Input: part model. Units: mm. Frame: model coordinates. Round coordinates to 2 decimals unless told otherwise and drop trailing zeros. Order: outer loops, then holes, each group sorted by start corner. A loop starts at its lowest first (then second) coordinate and runs counter-clockwise, first axis right, second up.
Item 1: Cut plane B-B on y = -22.5. Output: boundary loops of the cut face in (x, z).
Item 2: Cut plane C-C on z = 4.5. Output: boundary loops of the cut face in (x, y), then the cut area to 3 significant figures.
Item 3: Cut plane A-A on z = 0. Output: boundary loops of the cut face in (x, y).
Item 4: Line query: L1, parallel to X at y = 3, z = 0; L2, parallel to Z at x = 0, y = 16.5; L3, parallel to Y at x = 0, z = -7.85. Output: solid intervals per line, ascending.
Item 5: Cut plane D-D on x = 3. Output: boundary loops of the cut face in (y, z), then the cut area to 3 significant figures.
Item 6: First-contact query: pin 1 (0.7 mm diameter, centred on x = -8, y = 3.5, fed in from +Z); pin 2 (1.8 mm diameter, centred on x = -8, y = 9.5, fed in from -Z); pin 3 (6 mm diameter, centred on x = -4.5, y = -16, fed in from -Z). Flat tips, straight axial feed; report the tip coordinate or a pass-through.
```python
from build123d import *

# Parameters (mm, degrees)
SKETCH1_R               = 11
SKETCH1_R_2             = 7
BOSS_EXTRUDE1_DEPTH     = 36.75
SKETCH2_R               = 1.25
CUT_EXTRUDE1_DEPTH      = 10
CIRPATTERN1_COUNT       = 2
CIRPATTERN1_ANGLE       = 90
CUT_EXTRUDE2_DEPTH      = 76.128223855
CUT_EXTRUDE2_DEPTH_BACK = 76.128223855


with BuildPart() as part:
    # Sketch1 → Boss-Extrude1 (new, symmetric)
    with BuildSketch(Plane(origin=(0, 0, 0), x_dir=(1, 0, 0), z_dir=(0, 1, 0))):
        with Locations(Location((0, 0, 0), (0, 0, 270))):
            Circle(SKETCH1_R)
        with Locations(Location((0, 0, 0), (0, 0, 270))):
            Circle(SKETCH1_R_2, mode=Mode.SUBTRACT)
    extrude(amount=BOSS_EXTRUDE1_DEPTH, both=True)

    # Sketch2 → Cut-Extrude1 (cut)
    with BuildSketch(Plane(origin=(0, 0, -11), x_dir=(-1, 0, 0), z_dir=(0, 0, -1))):
        with Locations(Location((0, 29.75, 0), (0, 0, 90))):
            Circle(SKETCH2_R)
    cut_extrude1 = extrude(amount=-CUT_EXTRUDE1_DEPTH, mode=Mode.SUBTRACT)

    # CirPattern1: Cut-Extrude1 ×2 about axis
    cirpattern1_axis = Axis((0, 36.75, 0), (0, -1, 0))
    for i in range(1, CIRPATTERN1_COUNT):
        add(cut_extrude1.rotate(cirpattern1_axis, i * CIRPATTERN1_ANGLE / (CIRPATTERN1_COUNT - 1)), mode=Mode.SUBTRACT)

    # Sketch4 → Cut-Extrude2 (cut, two sides: drawn at the far end of the back side and taken through both)
    with BuildSketch(Plane(origin=(0, 36.75, 0), x_dir=(1, 0, 0), z_dir=(0, 1, 0)).offset(-CUT_EXTRUDE2_DEPTH_BACK)):
        with BuildLine():
            ThreePointArc((-6.565325544, 2.428271092), (-6.551935139, 2.464172464), (-6.538348415, 2.5))
            Line((-6.538348415, 2.5), (-8.738348415, 2.5))
            Line((-8.738348415, 2.5), (-8.738348415, -2.5))
            Line((-8.738348415, -2.5), (-6.538348415, -2.5))
            ThreePointArc((-6.538348415, -2.5), (-6.999895128, -0.038317104), (-6.565325544, 2.428271092))
        make_face()
    extrude(amount=CUT_EXTRUDE2_DEPTH + CUT_EXTRUDE2_DEPTH_BACK, mode=Mode.SUBTRACT)


solid = part.part
```
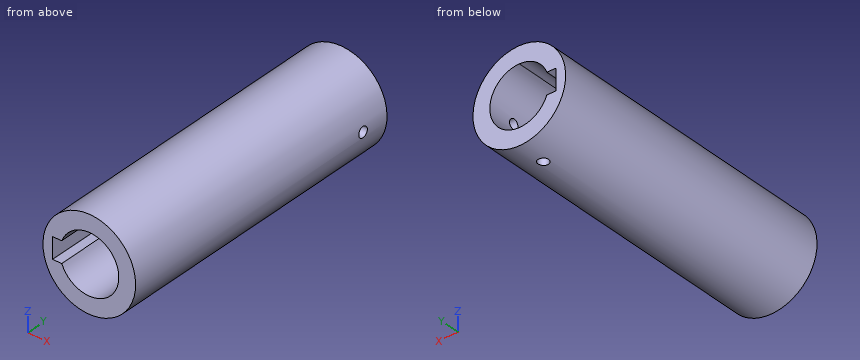
From the geometry:
1. outline: circle Ø22 at (0, 0); hole (-8.74, -2.5) - (-6.54, -2.5) arc R7 ccw (long way) to (-6.54, 2.5) - (-8.74, 2.5) - close
2. outline: (-10.04, -36.75) - (-5.36, -36.75) - (-5.36, 36.75) - (-10.04, 36.75) - close; (5.36, -36.75) - (10.04, -36.75) - (10.04, 36.75) - (5.36, 36.75) - close
2. area: 687 mm2
3. outline: (-11, -36.75) - (-8.74, -36.75) - (-8.74, 36.75) - (-11, 36.75) - close; (7, -36.75) - (11, -36.75) - (11, 28.5) - (7, 28.5) - close; (7, 31) - (11, 31) - (11, 36.75) - (7, 36.75) - close
4. L1: x = -11 to -8.74, 7 to 11
4. L2: z = -11 to -7, 7 to 11
4. L3: y = -36.75 to 28.5, 31 to 36.75
5. outline: (-36.75, -10.58) - (36.75, -10.58) - (36.75, -6.32) - (-36.75, -6.32) - close; (-36.75, 6.32) - (36.75, 6.32) - (36.75, 10.58) - (-36.75, 10.58) - close
5. area: 626 mm2
6. pin 1: stops at z = 7.9
6. pin 2: stops at z = -8.4
6. pin 3: stops at z = -10.9
